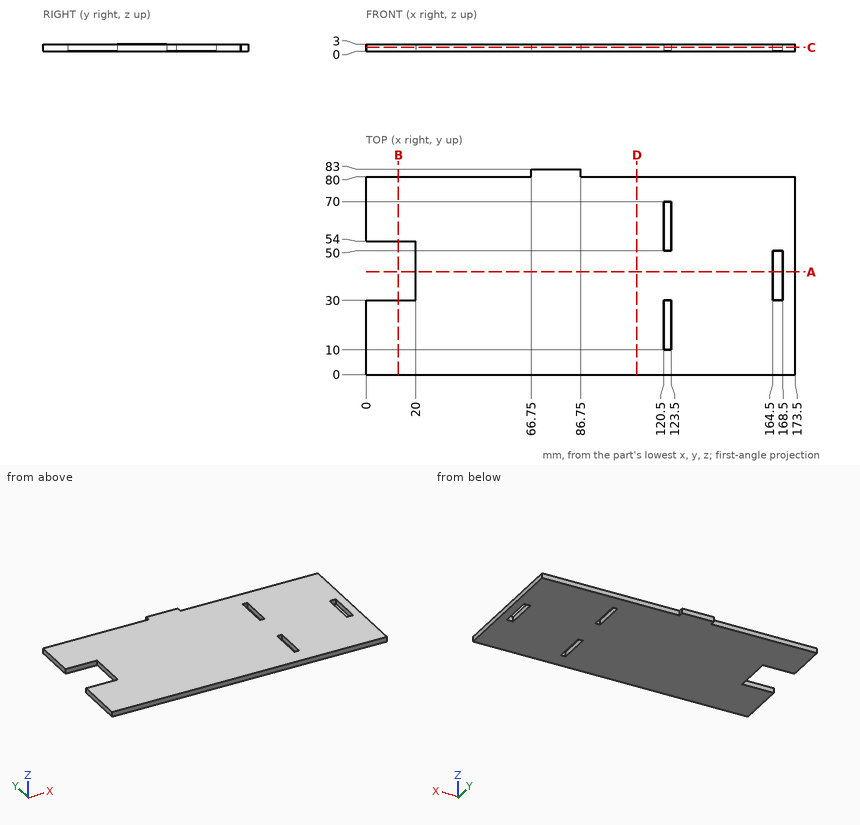
Verification items for this drawing (mm, ordinates from the low corner). Round coordinates to 2 decimals unless told otherwise and drop trailing zeros. Order: outer loops, then holes, each group sorted by start corner. A loop starts at its lowest first (then second) coordinate and runs counter-clockwise, first axis right, second up. Notation, with made-up numbers: M 51.25,-32 L 70.25,-32 A12 ccw 70.25,-26 Z; hole C 32,86 d7. An arc over 180 degrees is marked long. Answer in a Markdown table with one row per item. Add a question column.
Item 1: Sectioned sample at A-A, the plane y = 41.5. Enter the section's corners in (x, z).
Item 2: Sectioned sample at D-D, the plane x = 109.5. Enter the section's corners in (y, z).
Item 3: Depth check by flat-ended pin: pin 1 Ø0.9 at (y, z) = (81, 2) entering from -X; pin 2 Ø1.5 at (y, z) = (59, 1.5) entering from -X; pin 3 Ø0.9 at (x, z) = (125.5, 2) entering from +Y; pin 4 Ø0.9 at (y, z) = (42, 2) entering from -X. Enter the tip coordinate at first touch or a pass-through.
Item 4: Sectioned sample at C-C, the plane z = 1.6. Enter the section's corners in (x, y), plus the area to 3 significant figures.
Item 5: Sectioned sample at B-B, the plane x = 13. Enter the section's corners in (y, z), plus the area to 3 significant figures.
Item 6: Material ranges on L1, parallel to Y at x = 123, z = 1.1; L2, parallel to X at y = 62.5, z = 0.5; L3, parallel to X at y = 38, z = 1.65, recorded low to high. Write a range as [from, to].
Filled in:
| question | item | result |
|---|---|---|
| 1 | outline | M 20,0 L 164.5,0 L 164.5,3 L 20,3 Z; M 168.5,0 L 173.5,0 L 173.5,3 L 168.5,3 Z |
| 2 | outline | M 0,0 L 80,0 L 80,3 L 0,3 Z |
| 3 | pin 1 | stops at x = 66.75 |
| 3 | pin 2 | stops at x = 0 |
| 3 | pin 3 | stops at y = 80 |
| 3 | pin 4 | stops at x = 20 |
| 4 | outline | M 0,0 L 173.5,0 L 173.5,80 L 86.75,80 L 86.75,83 L 66.75,83 L 66.75,80 L 0,80 L 0,54 L 20,54 L 20,30 L 0,30 Z; hole M 120.5,10 L 123.5,10 L 123.5,30 L 120.5,30 Z; hole M 120.5,50 L 123.5,50 L 123.5,70 L 120.5,70 Z; hole M 164.5,30 L 168.5,30 L 168.5,50 L 164.5,50 Z |
| 4 | area | 13,300 mm² |
| 5 | outline | M 0,0 L 30,0 L 30,3 L 0,3 Z; M 54,0 L 80,0 L 80,3 L 54,3 Z |
| 5 | area | 168 mm² |
| 6 | L1 | y = [0, 10], [30, 50], [70, 80] |
| 6 | L2 | x = [0, 120.5], [123.5, 173.5] |
| 6 | L3 | x = [20, 164.5], [168.5, 173.5] |
